Geometry: final body of the model. Coordinates: model frame, mm. A direction names the side the tool comes from. Give positions to 0.01 mm unless a question says otherwise; leave off trailing zeros. Loops run counter-clockwise (first coordinate to the right, second up) from the corner with the lowest first, then second, coordinate; pieces in that order, holes last.
```python
from build123d import *

# Parameters (mm, degrees)
SKETCH1_R           = 18.75
BOSS_EXTRUDE1_DEPTH = 29
SKETCH3_R           = 1.99
BOSS_EXTRUDE4_DEPTH = 3
CHAMFER1_SIZE       = 5
SKETCH4_R           = 1.99
BOSS_EXTRUDE5_DEPTH = 1
SKETCH5_R           = 1.5
CUT_EXTRUDE1_DEPTH  = 1
CIRPATTERN1_COUNT   = 4


with BuildPart() as part:
    # Sketch1 → Boss-Extrude1 (new body)
    with BuildSketch(Plane.XY):
        Circle(SKETCH1_R)
    extrude(amount=BOSS_EXTRUDE1_DEPTH)

    # Sketch3 → Boss-Extrude4 (add)
    with BuildSketch(Plane.XY.offset(29)):
        Circle(SKETCH3_R)
    extrude(amount=BOSS_EXTRUDE4_DEPTH)

    # Chamfer1
    chamfer1_edges = [part.edges().sort_by_distance(p)[0] for p in [
        (-18.75, 0, 0),
        (-18.75, 0, 29),
    ]]
    chamfer(chamfer1_edges, length=CHAMFER1_SIZE)

    # Sketch4 → Boss-Extrude5 (add)
    with BuildSketch(Plane(origin=(0, 0, 0), x_dir=(-1, 0, 0), z_dir=(0, 0, -1))):
        Circle(SKETCH4_R)
    extrude(amount=BOSS_EXTRUDE5_DEPTH)

    # Sketch5 → Cut-Extrude1 (cut)
    with BuildSketch(Plane(origin=(0, 0, 0), x_dir=(-1, 0, 0), z_dir=(0, 0, -1))):
        with Locations((0, 8)):
            Circle(SKETCH5_R)
    cut_extrude1 = extrude(amount=-CUT_EXTRUDE1_DEPTH, mode=Mode.SUBTRACT)

    # CirPattern1: Cut-Extrude1 ×4 about axis
    cirpattern1_axis = Axis((0, 0, 0), (0, 0, 1))
    for i in range(1, CIRPATTERN1_COUNT):
        add(cut_extrude1.rotate(cirpattern1_axis, i * 360 / CIRPATTERN1_COUNT), mode=Mode.SUBTRACT)


solid = part.part
```
Q1. Section query C-C, the plane z = 20. Return loops of the section in (x, y).
Q2. Mould query, pull axis X, two halves, no side actions, for faces 4 (the face through (-8, 0, 1)), 5 (the face through (0, -3, 29)), 6 (the face through (-11.104, -8.514, 28.757)). Classes: +X half, -X half, draft (parallel to the pull), parting line (faces both ways), or undercut.
Q3. Reachability of faces 1 (the face through (0, -8, 1)), 2 (the face through (0, 0, -1)), 3 (the face through (-0.259, 1.973, 30.479)) from +Z, -Z, +X, -X, +Y, -Y: full face, straight path, thin tool, end or side. Return the list, or none.
Q4. Section query D-D, the plane z = 3.5. Return loops of the section in (x, y), and give its area (3 significant figures).
Q5. Pin query (flat end, axial travel): pin 1 Ø5 at (x, y) = (0, -8) entering from +Z; pin 2 Ø3.5 at (x, y) = (-0.5, 8) entering from -Z; pin 3 Ø1.5 at (x, z) = (-7.5, 26) entering from +Y; pin 4 Ø8 at (x, y) = (3, 4.5) entering from -Z. Return the tip coordinate at first contact, or that it passes through.
Q6. Material intervals for probe 1 along Y at (x, z) = (0, 0.4); probe 2 along Z at (x, y) = (0.5, 13.5); probe 3 along Y at (x, z) = (0, 0.5), sorted ascending.
Q7. Section query A-A, the plane y = 0. Return loops of the section in (x, z), and give its area (3 significant figures).
Resolved:
1. outline: circle Ø37.5 at (0, 0)
2. face 4: undercut
2. face 5: draft
2. face 6: parting line
3. face 1: -Z
3. face 2: -Z, +X, -X, +Y, -Y
3. face 3: +Z
4. outline: circle Ø34.5 at (0, 0)
4. area: 935 mm2
5. pin 1: stops at z = 29
5. pin 2: stops at z = 0
5. pin 3: stops at y = 15.88
5. pin 4: stops at z = -1
6. probe 1: y = -14.15 to -9.5, -6.5 to 6.5, 9.5 to 14.15
6. probe 2: z = 0 to 29
6. probe 3: y = -14.25 to -9.5, -6.5 to 6.5, 9.5 to 14.25
7. outline: (-18.75, 5) - (-13.75, 0) - (-9.5, 0) - (-9.5, 1) - (-6.5, 1) - (-6.5, 0) - (-1.99, 0) - (-1.99, -1) - (1.99, -1) - (1.99, 0) - (6.5, 0) - (6.5, 1) - (9.5, 1) - (9.5, 0) - (13.75, 0) - (18.75, 5) - (18.75, 24) - (13.75, 29) - (1.99, 29) - (1.99, 32) - (-1.99, 32) - (-1.99, 29) - (-13.75, 29) - (-18.75, 24) - close
7. area: 1,050 mm2
